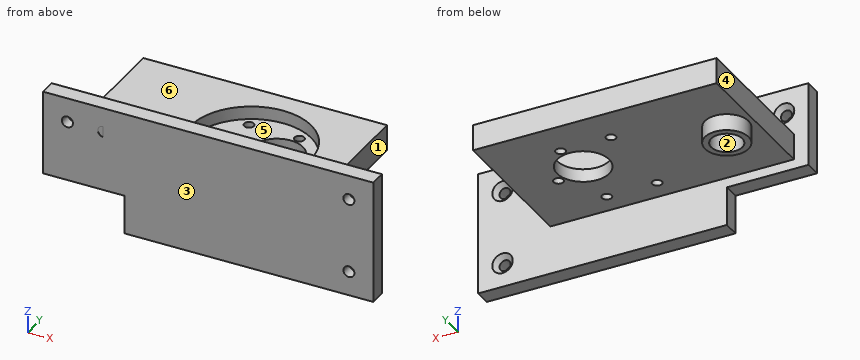
from build123d import *

# Parameters (mm, degrees)
SKETCH3_W                                       = 57.15
SKETCH3_H                                       = 50
BOSS_EXTRUDE1_DEPTH                             = 8
SKETCH3_3_R                                     = 1.5
SKETCH3_3_R_2                                   = 8
CUT_EXTRUDE2_DEPTH                              = 10
SKETCH4_R                                       = 18.5
CUT_EXTRUDE3_DEPTH                              = 4
BOSS_EXTRUDE2_DEPTH                             = 15
BOSS_EXTRUDE2_DEPTH_BACK                        = 23
SKETCH6_W                                       = 101.6
SKETCH6_H                                       = 5
CSK_FOR_M3_FLAT_HEAD_MACHINE_SCREW1_D           = 3.4
CSK_FOR_M3_FLAT_HEAD_MACHINE_SCREW1_CSINK_D     = 6.3
CSK_FOR_M3_FLAT_HEAD_MACHINE_SCREW1_CSINK_ANGLE = 90
CUT_EXTRUDE6_REACH                              = 555.432
SKETCH16_R                                      = 1.7
CUT_EXTRUDE7_REACH                              = 73.656
SKETCH17_W                                      = 25.08228791
SKETCH17_H                                      = 11.980848154
SKETCH18_W                                      = 17.78
SKETCH18_H                                      = 8
BOSS_EXTRUDE3_DEPTH                             = 45
SKETCH13_R                                      = 6.7056
SKETCH13_R_2                                    = 4.8006
BOSS_EXTRUDE4_DEPTH                             = 5.08
CUT_EXTRUDE8_START                              = -5.08
SKETCH19_R                                      = 4.8006
CUT_EXTRUDE8_DEPTH                              = 5.08


with BuildPart() as part:
    # Sketch3 → Boss-Extrude1 (new body)
    with BuildSketch(Plane.XY):
        with Locations((0, 25)):
            Rectangle(SKETCH3_W, SKETCH3_H)
    extrude(amount=BOSS_EXTRUDE1_DEPTH)

    # Sketch3<3> → Cut-Extrude2 (cut)
    with BuildSketch(Plane.XY):
        with Locations(Location((-7.75, 38.423393759, 0), (0, 0, 180))):
            Circle(SKETCH3_3_R)
        with Locations(Location((7.75, 38.423393759, 0), (0, 0, 180))):
            Circle(SKETCH3_3_R)
        with Locations(Location((-7.75, 11.576606241, 0), (0, 0, 180))):
            Circle(SKETCH3_3_R)
        with Locations(Location((7.75, 11.576606241, 0), (0, 0, 180))):
            Circle(SKETCH3_3_R)
        with Locations(Location((15.5, 25, 0), (0, 0, 180))):
            Circle(SKETCH3_3_R)
        with Locations(Location((6.062177825, 28.499999999, 0), (0, 0, 180))):
            Circle(SKETCH3_3_R_2)
    extrude(amount=CUT_EXTRUDE2_DEPTH, mode=Mode.SUBTRACT)

    # Sketch4 → Cut-Extrude3 (cut)
    with BuildSketch(Plane.XY.offset(8)):
        with Locations((0, 25)):
            Circle(SKETCH4_R)
    extrude(amount=-CUT_EXTRUDE3_DEPTH, mode=Mode.SUBTRACT)

    # Sketch6 → Boss-Extrude2 (add, two sides: drawn at the far end of the back side and taken through both)
    with BuildSketch(Plane.XY.offset(8).offset(-BOSS_EXTRUDE2_DEPTH_BACK)):
        with Locations((0, 2.5)):
            Rectangle(SKETCH6_W, SKETCH6_H)
    extrude(amount=BOSS_EXTRUDE2_DEPTH + BOSS_EXTRUDE2_DEPTH_BACK)

    # CSK for M3 Flat Head Machine Screw1 (through all)
    with Locations(Plane(origin=(0, 5, 0), x_dir=(1, 0, 0), z_dir=(0, 1, 0))):
        with Locations((-43.3, 7.5), (-43.3, -15.5), (43.3, -15.5), (43.3, 7.5)):
            CounterSinkHole(CSK_FOR_M3_FLAT_HEAD_MACHINE_SCREW1_D / 2, CSK_FOR_M3_FLAT_HEAD_MACHINE_SCREW1_CSINK_D / 2, counter_sink_angle=CSK_FOR_M3_FLAT_HEAD_MACHINE_SCREW1_CSINK_ANGLE)

    # Sketch16 → Cut-Extrude6 (cut, up to next)
    with BuildSketch(Plane(origin=(-499.248949842, 16.821159134, -28.308871479), x_dir=(0.050830850863696445, -0.0009181581696577921, 0.9987068546806156), z_dir=(0.036090886531912156, 0.9993480899541041, -0.0009181581696584951)), mode=Mode.PRIVATE) as cut_extrude6_sk1:
        with Locations((67.5, 464.499999998)):
            Circle(SKETCH16_R)
    cut_extrude6_tool1 = extrude(cut_extrude6_sk1.sketch, amount=-CUT_EXTRUDE6_REACH, mode=Mode.PRIVATE) & part.part
    # Sketch16 → Cut-Extrude6 (cut, up to next)
    with BuildSketch(Plane(origin=(-499.248949842, 16.821159134, -28.308871479), x_dir=(0.050830850863696445, -0.0009181581696577921, 0.9987068546806156), z_dir=(0.036090886531912156, 0.9993480899541041, -0.0009181581696584951)), mode=Mode.PRIVATE) as cut_extrude6_sk2:
        with Locations((44.5, 464.499999998)):
            Circle(SKETCH16_R)
    cut_extrude6_tool2 = extrude(cut_extrude6_sk2.sketch, amount=-CUT_EXTRUDE6_REACH, mode=Mode.PRIVATE) & part.part
    add(cut_extrude6_tool1.solids().sort_by_distance((-32.221346, -0.005033, 15.492911))[0], mode=Mode.SUBTRACT)
    add(cut_extrude6_tool2.solids().sort_by_distance((-33.390455, 0.016084, -7.477347))[0], mode=Mode.SUBTRACT)

    # Sketch17 → Cut-Extrude7 (cut, up to next)
    with BuildSketch(Plane(origin=(0, 5, 0), x_dir=(1, 0, 0), z_dir=(0, 1, 0)), mode=Mode.PRIVATE) as cut_extrude7_sk1:
        with Locations((-38.258856045, 9.009575923)):
            Rectangle(SKETCH17_W, SKETCH17_H)
    cut_extrude7_tool1 = extrude(cut_extrude7_sk1.sketch, amount=-CUT_EXTRUDE7_REACH, mode=Mode.PRIVATE) & part.part
    add(cut_extrude7_tool1.solids().sort_by_distance((-38.258856, 5, -9.009576))[0], mode=Mode.SUBTRACT)

    # Sketch18 → Boss-Extrude3 (add)
    with BuildSketch(Plane(origin=(0, 5, 0), x_dir=(1, 0, 0), z_dir=(0, 1, 0))):
        with Locations((-37.465, -4)):
            Rectangle(SKETCH18_W, SKETCH18_H)
    extrude(amount=BOSS_EXTRUDE3_DEPTH)

    # Sketch13 → Boss-Extrude4 (add)
    with BuildSketch(Plane(origin=(0, 0, 0), x_dir=(-1, 0, 0), z_dir=(0, 0, -1))):
        with Locations((38.117822207, 28.499999999)):
            Circle(SKETCH13_R)
        with Locations((38.117822207, 28.499999999)):
            Circle(SKETCH13_R_2, mode=Mode.SUBTRACT)
    extrude(amount=BOSS_EXTRUDE4_DEPTH)

    # Sketch19 → Cut-Extrude8 (cut)
    with BuildSketch(Plane(origin=(0, 0, 0), x_dir=(-1, 0, 0), z_dir=(0, 0, -1)).offset(CUT_EXTRUDE8_START)):
        with Locations((38.117822207, 28.499999999)):
            Circle(SKETCH19_R)
    extrude(amount=CUT_EXTRUDE8_DEPTH, mode=Mode.SUBTRACT)


solid = part.part
The listing builds one solid part. Answer for the finished solid, in the listing's coordinates (mm). Face numbers are marked on the shaded views. A direction names the side the tool comes from. Coordinates: 2 decimals unless noted, no trailing zeros. Write each loop counter-clockwise with the first axis right and the second up, starting at its lowest first coordinate (ties: lowest second). Pieces come first, ordered by that corner, then holes. Notation, with made-up numbers: (-22.5, -11) - (4.5, -11) arc R20 cw to (4.5, 10) - close; hole circle Ø3 at (-35.75, -23.75). An arc over 180 degrees is marked (long way). Return JSON: item names as keys, results as strings.
1. Which of the six approach directions +Z, -Z, +X, -X, +Y, -Y give full straight-line access (tool end or side, diameter ignored) to the marked faces 4, 5 and 6?
Final values:
{"face 4": "+Z, -Z, -X, +Y", "face 5": "+Z", "face 6": "+Z, +X, -X, +Y"}
2. The part is cut by section A-A on x = 43.3. Determine the outline of the cut face in (y, z), then the cut area to 3 significant figures.
Final values:
{"outline": "(0, -15) - (5, -15) - (5, -10.65) - (3.55, -9.2) - (0, -9.2) - close; (0, -5.8) - (3.55, -5.8) - (5, -4.35) - (5, 12.35) - (3.55, 13.8) - (0, 13.8) - close; (0, 17.2) - (3.55, 17.2) - (5, 18.65) - (5, 23) - (0, 23) - close", "area": "152 mm^2"}
3. For a pull along X with two mould halves and no side action, classify the marked faces 1, 2 and 3 as +X half, -X half, draft (parallel to the pull), parting line (faces both ways), or undercut.
Final values:
{"face 1": "+X half", "face 2": "undercut", "face 3": "draft"}
4. Each of these flat-tipped pins is pushed along its axis until it touches: pin 1 Ø6 at (x, y) = (-38.12, 28.5) entering from +Z; pin 2 Ø5 at (x, y) = (-7.75, 38.42) entering from -Z; pin 3 Ø4 at (x, z) = (43.3, -7.5) entering from +Y. Where does it stop, or does it pass through?
Final values:
{"pin 1": "z = 8", "pin 2": "z = 0", "pin 3": "y = 3.85"}
5. The part is cut by section C-C on x = 0. Determine the outline of the cut face in (y, z), then the cut area to 3 significant figures.
Final values:
{"outline": "(0, -15) - (5, -15) - (5, 0) - (23.28, 0) - (23.28, 4) - (6.5, 4) - (6.5, 8) - (5, 8) - (5, 23) - (0, 23) - close; (33.72, 0) - (50, 0) - (50, 8) - (43.5, 8) - (43.5, 4) - (33.72, 4) - close", "area": "360 mm^2"}
6. The part is cut by section B-B on y = 30.5. Determine the outline of the cut face in (x, z) (3 decimals).
Final values:
{"outline": "(-46.355, 0) - (-44.518, 0) - (-44.518, -5.08) - (-42.482, -5.08) - (-42.482, 5.08) - (-33.754, 5.08) - (-33.754, -5.08) - (-31.717, -5.08) - (-31.717, 0) - (-1.684, 0) - (-1.684, 4) - (-17.664, 4) - (-17.664, 8) - (-46.355, 8) - close; (13.808, 0) - (28.575, 0) - (28.575, 8) - (17.664, 8) - (17.664, 4) - (13.808, 4) - close"}
7. The part is cut by section D-D on y = 15. Determine the outline of the cut face in (x, z) (3 decimals), then the cut area to 3 significant figures.
Final values:
{"outline": "(-46.355, 0) - (28.575, 0) - (28.575, 8) - (15.564, 8) - (15.564, 4) - (-15.564, 4) - (-15.564, 8) - (-46.355, 8) - close", "area": "475 mm^2"}
8. Consider line 1 along Z through (x, y) = (43.3, 1.2); line 2 along Y through (x, z) = (-7.75, 3.2); line 3 along X through (y, z) = (1.6, 15.5). Determine where each line is inside the solid, lowest interval first.
Final values:
{"line 1": "-15 to -9.2, -5.8 to 13.8, 17.2 to 23", "line 2": "0 to 10.08, 13.08 to 36.92, 39.92 to 50", "line 3": "-50.8 to -45, -41.6 to 41.6, 45 to 50.8"}
